Source: CAD feature listing. Evaluate the final solid. Frame: model axes, mm. Round coordinates to 2 decimals unless told otherwise and drop trailing zeros. Loops run counter-clockwise (first coordinate to the right, second up) from the corner with the lowest first, then second, coordinate; pieces in that order, holes last. Notation, with made-up numbers: (-25, 67.5) - (-8, 67.5) arc R18 ccw to (-8, 77.5) - close; hole circle Ø8 at (78.25, -11). An arc over 180 degrees is marked (long way). One line per question, with ' | ' between items.
Autodesk Inventor part; units mm, degrees
ref_plane "YZ Plane" through (0, 0, 0) normal (1, 0, 0) x (0, 1, 0)
ref_plane "XZ Plane" through (0, 0, 0) normal (0, 1, 0) x (-1, 0, 0)
ref_plane "XY Plane" through (0, 0, 0) normal (0, 0, 1) x (1, 0, 0)
sketch "Sketch1" plane through (0, 0, 0) normal (0, 0, 1) x (1, 0, 0)
  line L0 (1200, 2950) -> (-1200, 2950)
  line L1 (-1200, 2950) -> (-1200, 0)
  line L2 (-1200, 0) -> (1200, 0)
  line L3 (1200, 0) -> (1200, 2950)
  line L4 (1150, 2950) -> (1150, 0)
  line L5 (-1150, 0) -> (-1150, 2950) construction
  line L6 (0, 2950) -> (0, 50) construction
  line L7 (-1100, 200) -> (-950, 50)
  line L8 (-1200, 100) -> (-1100, 100)
  line L9 (-1100, 100) -> (-1100, 0)
  line L10 (-1100, 200) -> (-1150, 2950)
  arc A0 (-1100.4545, 224.9959) -> (-1082.3223, 182.3223) centre (-1100, 200) ccw
  arc A1 (-1082.3223, 182.3223) -> (-1100.4545, 224.9959) centre (-1100, 200) ccw construction
  line L11 (-1200, 255) -> (-1101, 255) construction
  line L12 (0, 50) -> (-950, 50)
  line L13 (0, 50) -> (0, 0)
  line L14 (1505.3449, -225.894) -> (355.3449, -225.894)
  line L15 (-1200, 245) -> (-1100.8182, 245)
  line L16 (-1200, 2900) -> (-1149.0909, 2900)
  dimension "d3" = 2400
  dimension "d4" = 2950
  dimension "d5" = 50
  dimension "d6" = 100
  dimension "d7" = 50
  dimension "d9" = 135
  dimension "d10" = 950
  dimension "d11" = 1150
  dimension "d12" = 136.042
  dimension "d13" = 50
  dimension "d14" = 100
  dimension "d15" = 212.132
  dimension "d17" = 55
  dimension "d20" = 200
  dimension "d50" = 2705
  dimension "d53" = 50
extrude "Plate1" add sketch "Sketch1" along normal blind 3 contours L10 L15 L1 L16
sketch "Sketch2" plane through (0, 0, 3) normal (0, 0, 1) x (1, 0, 0)
  line L0 (-1149.0909, 2900) -> (-1100.8182, 245)
  line L1 (-1200, 245) -> (-1200, 2900)
  line L2 (-1100.8182, 245) -> (-1150, 2950)
  line L3 (-1158.8362, 1267.3142) -> (-1158.778, 1264.1148)
  line L4 (-1158.778, 1264.1148) -> (-1119.3606, 1264.8314) construction
  line L5 (-1150, 2950) -> (-1100.8182, 245)
  line L6 (-1158.778, 1264.1148) -> (-1200, 1263.3653)
  line L7 (-1158.8362, 1267.3142) -> (-1200, 1266.5658)
  line L8 (-1200, 703.2727) -> (-1153.6813, 704.1149)
  line L9 (-1153.6813, 704.1149) -> (-1153.7395, 707.3144)
  line L10 (-1153.6813, 704.1149) -> (-1109.1804, 704.924) construction
  line L11 (-1153.7395, 707.3144) -> (-1200, 706.4732)
  line L12 (-1200, 1823.4578) -> (-1163.8614, 1824.1149)
  line L13 (-1163.8614, 1824.1149) -> (-1163.9196, 1827.3144)
  line L14 (-1163.9196, 1827.3144) -> (-1200, 1826.6584)
  line L15 (-1163.8614, 1824.1149) -> (-1129.5407, 1824.7389) construction
  line L16 (-1200, 2383.5504) -> (-1168.9515, 2384.1149)
  line L17 (-1168.9515, 2384.1149) -> (-1169.0097, 2387.3144)
  line L18 (-1168.9515, 2384.1149) -> (-1139.7208, 2384.6464) construction
  line L19 (-1169.0097, 2387.3144) -> (-1200, 2386.7509)
  line L20 (-1100.8182, 245) -> (-1200, 245)
  line L21 (-1200, 2900) -> (-1149.0909, 2900)
  point P0 (0, 0)
  dimension "d34" = 46.3264
  dimension "d36" = 41.2288
  dimension "d39" = 36.1445
  dimension "d42" = 31.0536
  dimension "d43" = 560
  dimension "d44" = 3.2
  dimension "d45" = 560
  dimension "d46" = 3.2
  dimension "d47" = 560
  dimension "d48" = 3.2
  dimension "d49" = 3.2
  dimension "d52" = 460
extrude "Extrusion1" cut sketch "Sketch2" against normal through all contours L19 L17 L16 L1 | L1 L11 L9 L8 | L14 L13 L12 L1 | L1 L7 L3 L6
equation "\"d11\" = d10 + d18"
equation "\"d14\" = d6"
equation "\"d43\" = Stringer1_step"
equation "\"d45\" = Stringer1_step"
equation "\"d47\" = Stringer1_step"
equation "\"d52\" = Stringer1_hight"
equation "\"d2\" = Thickness"
equation "\"BendReliefWidth\" = Thickness"
equation "\"BendReliefDepth\" = 0.5 * Thickness"
equation "\"CornerReliefSize\" = 4 * Thickness"
equation "\"MinimumRemnant\" = 2 * Thickness"
equation "\"TransitionRadius\" = BendRadius"
equation "\"JacobiRadiusSize\" = BendRadius"
equation "\"GapSize\" = Thickness"
equation "\"d18\" = d19"
properties part number "BSH 022 rib board" material "09g2s"
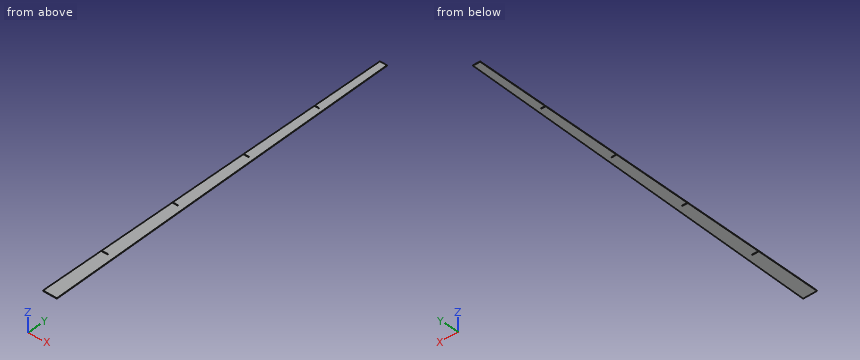
1. Material intervals for probe 1 along Y at (x, z) = (-1170, 1.15); probe 2 along Y at (x, z) = (-1178, 1.05); probe 3 along Y at (x, z) = (-1157, 0.3), sorted ascending.
Worked out:
probe 1: y = 245 to 703.82, 707.02 to 1263.91, 1267.11 to 1824, 1827.2 to 2384.1, 2387.3 to 2900 | probe 2: y = 245 to 703.67, 706.87 to 1263.77, 1266.97 to 1823.86, 1827.06 to 2383.95, 2387.15 to 2900 | probe 3: y = 245 to 704.05, 707.26 to 2900
2. Section query A-A, the plane z = 0.5. Return loops of the section in (x, y).
Worked out:
outline: (-1200, 245) - (-1100.82, 245) - (-1149.09, 2900) - (-1200, 2900) - (-1200, 2386.75) - (-1169.01, 2387.31) - (-1168.95, 2384.11) - (-1200, 2383.55) - (-1200, 1826.66) - (-1163.92, 1827.31) - (-1163.86, 1824.11) - (-1200, 1823.46) - (-1200, 1266.57) - (-1158.84, 1267.31) - (-1158.78, 1264.11) - (-1200, 1263.37) - (-1200, 706.47) - (-1153.74, 707.31) - (-1153.68, 704.11) - (-1200, 703.27) - close
3. Section query C-C, the plane y = 1988. Return loops of the section in (x, z).
Worked out:
outline: (-1200, 0) - (-1132.51, 0) - (-1132.51, 3) - (-1200, 3) - close
4. Contact query for a flat-ended pin moving along its axis: P1, Ø6, axis at x = -1155, y = 2348.5, coming from the -Z side. Output: stop coordinate, or through.
Worked out:
P1: stops at z = 0
5. Section query B-B, the plane y = 1714. Return loops of the section in (x, z), plus the area to 3 significant figures.
Worked out:
outline: (-1200, 0) - (-1127.53, 0) - (-1127.53, 3) - (-1200, 3) - close | area: 217 mm2
